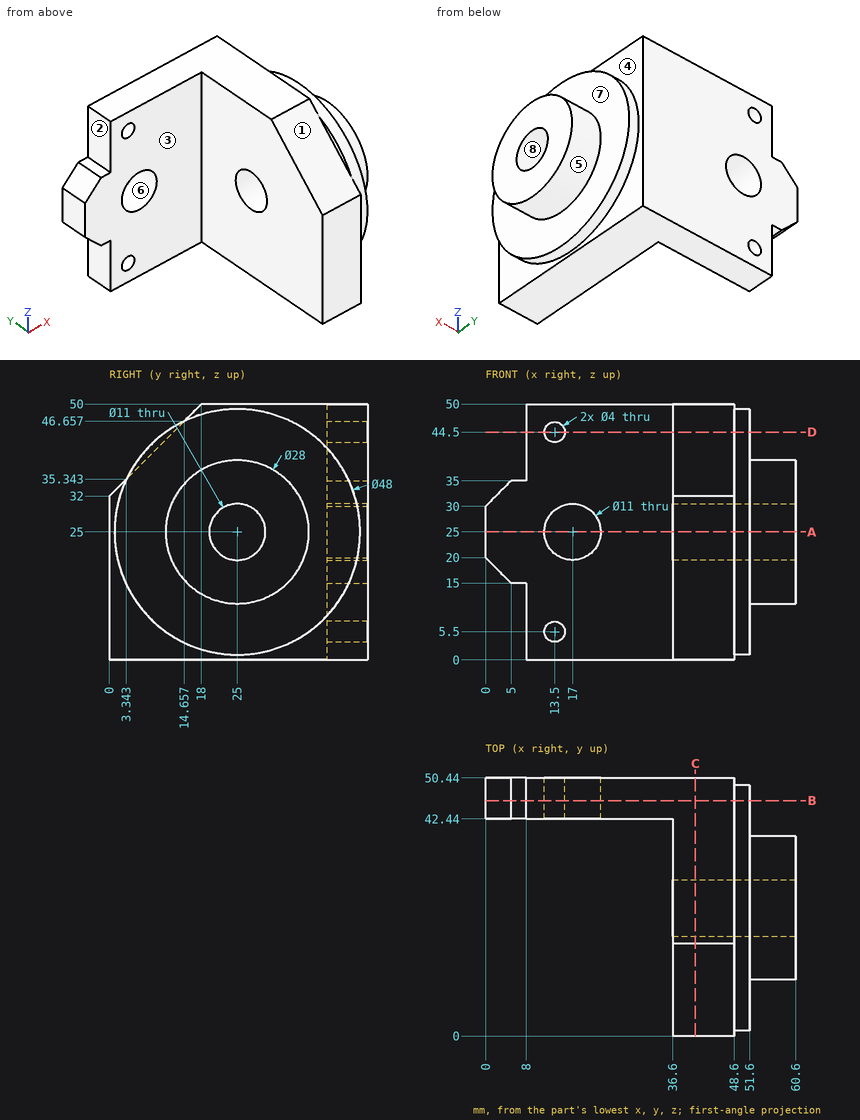
The figure shows three views and two pictorial views of one solid part (mm, origin at its lowest corner). Answer the questions. A direction names the side the tool comes from. Coordinates: 2 decimals unless noted, no trailing zeros. Loops run counter-clockwise (first coordinate to the right, second up) from the corner with the lowest first, then second, coordinate; pieces in that order, holes last. Notation, with made-up numbers: (77, -1) -> (110, -1) arc R7 cw to (110, 8) -> close; hole circle Ø6 at (75, 44.5). An arc over 180 degrees is marked (long way). Write item = value, one per line. Start each with the question number.
1) The mould has two halves that part along Z. Classify the marked faces 5, 6, 7 and 8: released by +Z, released by -Z, zero draft, split by the parting line, or undercut.
2) A cutting plane is placed at B-B (y = 46). Give the vertices of the cut face in (x, z), then the cut area to 3 significant figures.
3) Straight lines are drawn through the part: line 1 (Z direction, x = 13, y = 45) (1 decimal); line 2 (X direction, y = 49.25, z = 5.5); line 3 (X direction, y = 47, z = 44). For each, find the intervals that lie inside material, in ascending order. Write a range as from..to.
4) A tool of negligible diameter and unlimited length cuts with its end or side. For the marked faces 1, 2, 3 and 4, from which of +Z, -Z, +X, -X, +Y, -Y can it reach the whole face along a straight path? Write none if from no direction.
5) A cutting plane is placed at A-A (z = 25). Give the vertices of the cut face in (x, y), then the cut area to 3 significant figures.
6) Given pin 1 Ø6 at (y, z) = (6, 10) entering from -X; pin 2 Ø10 at (x, z) = (17, 25) entering from +Y; pin 3 Ø2.5 at (y, z) = (48, 7) entering from -X; pin 4 Ø3.5 at (x, y) = (6, 48) entering from +Z, each flat-ended and moving along its own axis, determine where each tip first touches the part or whether it passes through.
7) A cutting plane is placed at D-D (z = 44.5). Give the vertices of the cut face in (x, y).
8) A cutting plane is placed at C-C (x = 41). Give the vertices of the cut face in (y, z), then the cut area to 4 significant figures.
Responses:
q1.face_5 = split by the parting line
q1.face_6 = undercut
q1.face_7 = zero draft
q1.face_8 = undercut
q2.outline = (0, 20) -> (5, 15) -> (8, 15) -> (8, 0) -> (48.6, 0) -> (48.6, 13.38) -> (51.6, 13.38) -> (51.6, 36.62) -> (48.6, 36.62) -> (48.6, 50) -> (8, 50) -> (8, 35) -> (5, 35) -> (0, 30) -> close; hole circle Ø4 at (13.5, 5.5); hole circle Ø11 at (17, 25); hole circle Ø4 at (13.5, 44.5)
q2.area = 2,110 mm²
q3.line_1 = 0..3.6, 7.4..21.2, 28.8..42.6, 46.4..50
q3.line_2 = 8..11.5, 15.5..48.6
q3.line_3 = 8..11.56, 15.44..48.6
q4.face_1 = +Z, -X, -Y
q4.face_2 = +Z, -X, +Y, -Y
q4.face_3 = +Z, -Z, -X, -Y
q4.face_4 = +X
q5.outline = (0, 42.44) -> (11.5, 42.44) -> (11.5, 50.44) -> (0, 50.44) -> close; (22.5, 42.44) -> (36.6, 42.44) -> (36.6, 30.5) -> (60.6, 30.5) -> (60.6, 39) -> (51.6, 39) -> (51.6, 49) -> (48.6, 49) -> (48.6, 50.44) -> (22.5, 50.44) -> close; (36.6, 0) -> (48.6, 0) -> (48.6, 1) -> (51.6, 1) -> (51.6, 11) -> (60.6, 11) -> (60.6, 19.5) -> (36.6, 19.5) -> close
q5.area = 942 mm²
q6.pin_1 = 36.6
q6.pin_2 = through
q6.pin_3 = 8
q6.pin_4 = 35
q7.outline = (8, 42.44) -> (11.5, 42.44) -> (11.5, 50.44) -> (8, 50.44) -> close; (15.5, 42.44) -> (36.6, 42.44) -> (36.6, 12.5) -> (48.6, 12.5) -> (48.6, 11.01) -> (51.6, 11.01) -> (51.6, 38.99) -> (48.6, 38.99) -> (48.6, 50.44) -> (15.5, 50.44) -> close
q8.outline = (0, 0) -> (50.44, 0) -> (50.44, 50) -> (18, 50) -> (0, 32) -> close; hole circle Ø11 at (25, 25)
q8.area = 2,265 mm²
